Input: dimensioned drawing with shaded views. Units: mm. Origin: part minimum x, y, z. Round coordinates to 2 decimals unless told otherwise and drop trailing zeros. Loops run counter-clockwise (first coordinate to the right, second up) from the corner with the lowest first, then second, coordinate; pieces in that order, holes last.
1) Section A-A, the plane y = 10. Return loops of the section in (x, z).
2) Section D-D, the plane y = 15.25. Return loops of the section in (x, z), and give its area (3 significant figures).
3) Ray query, line 1 along Y through (x, z) = (15, 13.25); line 2 along Z through (x, y) = (21, 14.75); line 3 along X through (y, z) = (5.25, 10.5). Return the intervals inside material, ascending.
4) Section B-B, the plane z = 15. Return loops of the section in (x, y).
5) Section C-C, the plane x = 15. Return loops of the section in (y, z).
6) First-contact query: pin 1 (10 mm diameter, centred on y = 3, z = 3, fed in from -X). Flat tip, straight axial feed; report the tip coordinate or a pass-through.
7) Draft query along X for the marked faces 1, 2, 3 and 4. Return one class per face: pulls with the +X half, pulls with the -X half, needs draft (parallel to the pull), parting line crosses it, or undercut.
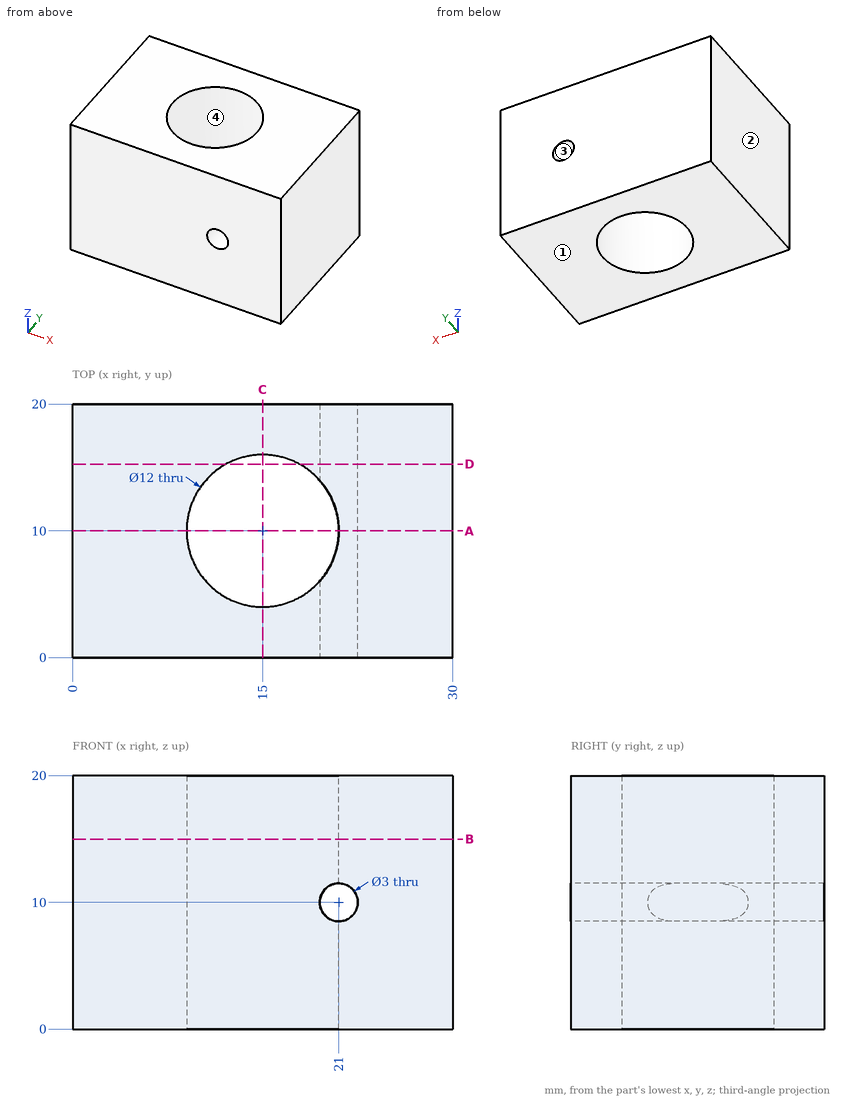
Final values:
1. outline: (0, 0) - (9, 0) - (9, 20) - (0, 20) - close; (21, 0) - (30, 0) - (30, 20) - (21, 20) - (21, 11.5) arc R1.5 cw to (21, 8.5) - close
2. outline: (0, 0) - (12.1, 0) - (12.1, 20) - (0, 20) - close; (17.9, 0) - (30, 0) - (30, 20) - (17.9, 20) - close; hole circle Ø3 at (21, 10)
2. area: 477 mm2
3. line 1: y = 0 to 4, 16 to 20
3. line 2: z = 0 to 8.5, 11.5 to 20
3. line 3: x = 0 to 11.33, 18.67 to 19.59, 22.41 to 30
4. outline: (0, 0) - (30, 0) - (30, 20) - (0, 20) - close; hole circle Ø12 at (15, 10)
5. outline: (0, 0) - (4, 0) - (4, 20) - (0, 20) - close; (16, 0) - (20, 0) - (20, 20) - (16, 20) - close
6. pin 1: stops at x = 0
7. face 1: needs draft
7. face 2: pulls with the -X half
7. face 3: undercut
7. face 4: undercut
